For this review, take the finished solid that the model builds, in its own axes (mm). A direction names the side the tool comes from. Give positions to 0.01 mm unless a question says otherwise; leave off trailing zeros. Write each loop counter-clockwise with the first axis right and the second up, starting at its lowest first coordinate (ties: lowest second). Pieces come first, ordered by that corner, then holes. Notation, with made-up numbers: M 75,40.25 L 80,40.25 A16 cw 80,45.25 Z; hole C 73.25,-32.75 d5. An arc over 180 degrees is marked long. Write item = value, one per line.
```python
from build123d import *

# Parameters (mm, degrees)
F1_DEPTH  = 20
F4_R      = 4.25
F5_DEPTH  = 20.001
F6_R      = 6.8
F6_R_2    = 4.25
F7_DEPTH  = 7
F10_R     = 8
F12_DEPTH = 20.001
F13_R     = 0.25


# Not quite as in the source:
# - a feature names something its author has since deleted; it is built from what else it names


with BuildPart() as f1:
    # F0 (on Right) → F1 (new body)
    with BuildSketch(Plane.YZ):
        Polygon((2.5455173281, 9.5), (0, 10.9696551146), (-9.5, 5.4848275573), (-9.5, -5.4848275573), (0, -10.9696551146), (2.5455173281, -9.5), (9.5, -5.4848275573), (9.5, 0), (9.5, 5.4848275573), align=None)
        Polygon((20, 9.5), (2.5455173281, 9.5), (9.5, 5.4848275573), (9.5, 0), (20, 0), align=None)
        Polygon((20, 0), (9.5, 0), (9.5, -5.4848275573), (2.5455173281, -9.5), (20, -9.5), align=None)
    extrude(amount=F1_DEPTH)

    # F4 (on face) → F5 (cut, through all)
    with BuildSketch(Plane(origin=(0, 0, 0), x_dir=(0, -1, 0), z_dir=(-1, 0, 0))):
        Circle(F4_R)
    extrude(amount=-F5_DEPTH, mode=Mode.SUBTRACT)


with BuildPart() as f7:
    # F6 (on face) → F7 (new body)
    with BuildSketch(Plane(origin=(0, 0, 0), x_dir=(0, -1, 0), z_dir=(-1, 0, 0))):
        with Locations((0.3292050309, 0)):
            Circle(F6_R)
        Circle(F6_R_2, mode=Mode.SUBTRACT)
        Circle(F6_R_2)
    extrude(amount=-F7_DEPTH)


with BuildPart() as f8_1:
    # F8: instance of F7
    add(f7.part.mirror(Plane(origin=(10, 5.820047307, 0), x_dir=(0, 1, 0), z_dir=(1, 0, 0))))


with BuildPart() as f1_1:
    add(f1.part)

    # F9: cut F7, F8_1
    add(f7.part, mode=Mode.SUBTRACT)
    add(f8_1.part, mode=Mode.SUBTRACT)

    # F10
    f10_edges = [f1_1.edges().sort_by_distance(p)[0] for p in [
        (10, 2.545517, -9.5),
        (10, 2.545517, 9.5),
    ]]
    fillet(f10_edges, radius=F10_R)

    # F11 (on face) → F12 (cut, through all)
    with BuildSketch(Plane.YZ.offset(20)):
        with BuildLine():
            Line((20, 0), (20, 2))
            ThreePointArc((20, 2), (18.5857864376, 1.4142135624), (18, 0))
            Line((18, 0), (20, 0))
        make_face()
        with BuildLine():
            ThreePointArc((18, 0), (18.5857864376, -1.4142135624), (20, -2))
            Line((20, -2), (20, 0))
            Line((20, 0), (18, 0))
        make_face()
        with BuildLine():
            ThreePointArc((20, -2), (21.4142135624, -1.4142135624), (22, 0))
            ThreePointArc((22, 0), (21.4142135624, 1.4142135624), (20, 2))
            Line((20, 2), (20, 0))
            Line((20, 0), (20, -2))
        make_face()
    extrude(amount=-F12_DEPTH, mode=Mode.SUBTRACT)

    # F13
    f13_edges = [f1_1.edges().sort_by_distance(p)[0] for p in [
        (10, -9.5, -5.484828),
        (10, -9.5, 5.484828),
        (10, 0, 10.969655),
        (10, 0, -10.969655),
    ]]
    fillet(f13_edges, radius=F13_R)


solid = f1_1.part
```
1. Insertion check: P1, Ø12, axis at y = -0.33, z = 0, coming from the -X side; P2, Ø7.5, axis at x = 13.5, y = 9, coming from the +Z side; P3, Ø4.5, axis at x = 10.5, y = 9.5, coming from the -Z side. Each pin has a flat end and moves straight along its axis. Give the tip position at first contact, or say it passes through.
Responses:
P1 = 7
P2 = 9.5
P3 = -9.5
2. For line 1 along Z through (x, y) = (10.05, 0); line 2 along X through (y, z) = (-2.25, 5.25); line 3 along Z through (x, y) = (7.75, 8.5), list the stretches that pass through material, from the lowest coordinate up. Write a range as from..to.
Responses:
line_1 = -10.93..-4.25, 4.25..10.93
line_2 = 7..13
line_3 = -9.5..9.5
3. We need section D-D, the plane y = -5.5. Write out the cut boundary in (x, z), then the cut area to 3 significant figures.
Responses:
outline = M 0,-7.79 L 20,-7.79 L 20,-4.42 L 13,-4.42 L 13,4.42 L 20,4.42 L 20,7.79 L 0,7.79 L 0,4.42 L 7,4.42 L 7,-4.42 L 0,-4.42 Z
area = 188 mm2
4. We need section A-A, the plane x = 14.25. Write out the cut boundary in (y, z) (3 decimals).
Responses:
outline = M -9.5,-5.34 A0.25 ccw -9.375,-5.557 L -0.125,-10.897 A0.25 ccw 0.125,-10.897 L 0.689,-10.572 A8 cw 4.689,-9.5 L 20,-9.5 L 20,-2 A2 cw 20,2 L 20,9.5 L 4.689,9.5 A8 cw 0.689,10.572 L 0.125,10.897 A0.25 ccw -0.125,10.897 L -9.375,5.557 A0.25 ccw -9.5,5.34 Z; hole C -0.329,0 d13.6
5. The part is to be moulded in two halves that separate along Y. For faces 5 (the face through (16.55, 1.14, -6.64)), 6 (the face through (10, 20, 6)), 7 (the face through (10, 12, -9.5)), say which applies: +Y half, -Y half, draft (parallel to the pull), parting line (faces both ways), or undercut.
Responses:
face_5 = undercut
face_6 = +Y half
face_7 = draft
6. Machinability: for faces 1 (the face through (9.9, -4.8, -8.2)), 2 (the face through (10, 12, 9.5)), 3 (the face through (13, -5, 0)), 4 (the face through (7, -5, 0)), which of the approach directions +Z, -Z, +X, -X, +Y, -Y give a long, thin tool a straight path to every point of the face, cutting with its end or side? Answer none if there is none.
Responses:
face_1 = -Z, +X, -X, -Y
face_2 = +Z, +X, -X, +Y
face_3 = +X
face_4 = -X
7. We need section B-B, the plane y = -2.25. Write out the cut boundary in (x, z).
Responses:
outline = M 0,-9.67 L 20,-9.67 L 20,-6.52 L 13,-6.52 L 13,-3.61 L 7,-3.61 L 7,-6.52 L 0,-6.52 Z; M 0,6.52 L 7,6.52 L 7,3.61 L 13,3.61 L 13,6.52 L 20,6.52 L 20,9.67 L 0,9.67 Z
8. We need section C-C, the plane z = 3.75. Write out the cut boundary in (x, y).
Responses:
outline = M 0,-9.5 L 20,-9.5 L 20,-6 L 13,-6 L 13,-2 L 7,-2 L 7,-6 L 0,-6 Z; M 0,5.34 L 7,5.34 L 7,2 L 13,2 L 13,5.34 L 20,5.34 L 20,20 L 0,20 Z
